Geometry check sheet. Reference: the model listing, model coordinates, mm. Face numbers are marked on the shaded views. A direction names the side the tool comes from. Give positions to 0.01 mm unless a question says otherwise; leave off trailing zeros. Loops run counter-clockwise (first coordinate to the right, second up) from the corner with the lowest first, then second, coordinate; pieces in that order, holes last. Notation, with made-up numbers: (76.25, 24.25) - (129.25, 24.25) arc R8 cw to (129.25, 30.25) - close; hole circle Ø8 at (36.25, -15). An arc over 180 degrees is marked (long way). Use a Markdown table: item, result. Add a question column.
1. Cross-section at A-A on z = 47. Enter the section's corners in (x, y), and give its area (3 significant figures).
2. Set-up check for the marked faces 1, 2, 3, 4 and 5: record each of +Z, -Z, +X, -X, +Y, -Y from which the full face is reachable in a straight line by a thin tool's end or side.
3. Depth check by flat-ended pin: P1, Ø3, axis at x = -51, y = 108.21, coming from the -Z side (3 decimals); P2, Ø4, axis at x = 31.5, z = 30, coming from the +Y side; P3, Ø10, axis at x = -39, z = 47, coming from the +Y side. Enter the tip coordinate at first touch or a pass-through.
4. Cross-section at B-B on x = 0. Enter the section's corners in (y, z), and give its area (3 significant figures).
5. Cross-section at C-C on z = 35.5. Enter the section's corners in (x, y).
6. Draft check along Y on the marked faces 6, 7 and 8. Enter one of: pulls with the +Y half, pulls with the -Y half, needs draft (parallel to the pull), parting line crosses it, or undercut.
7. Material ranges on L1, parallel to Y at x = 0, z = 2; L2, parallel to Y at x = 51, z = 4; L3, parallel to Z at x = 54.5, y = 77, recorded low to high.
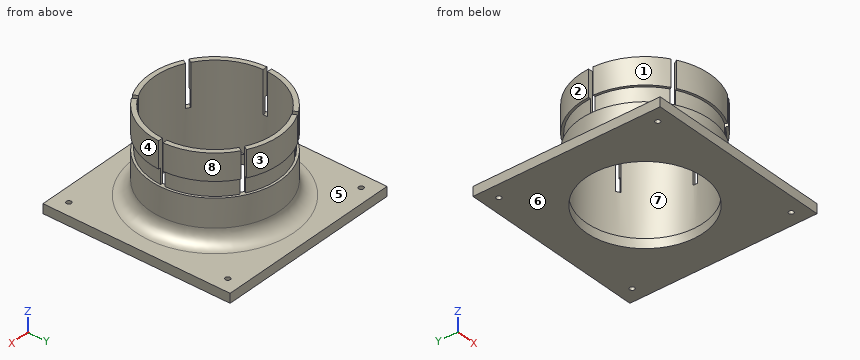
Autodesk Inventor part; units mm, degrees
ref_plane "Work Plane1" through (0, 57.2078, 33) normal (0, 0, 1) x (1, 0, 0)
ref_plane "YZ Plane" through (0, 0, 0) normal (1, 0, 0) x (0, 1, 0)
ref_plane "XZ Plane" through (0, 0, 0) normal (0, 1, 0) x (-1, 0, 0)
sketch "Sketch1" plane through (0, 0, 0) normal (0, 0, 1) x (1, 0, 0)
  circle A0 centre (-51, -113.7922) radius 1.55
  circle A1 centre (51, -113.7922) radius 1.55
  circle A2 centre (-51, 108.2078) radius 1.55
  circle A3 centre (51, 6.2078) radius 1.55
  circle A4 centre (51, 108.2078) radius 1.55
  circle A5 centre (-51, 6.2078) radius 1.55
  circle A6 centre (51, -11.7922) radius 1.55
  circle A7 centre (-51, -11.7922) radius 1.55
  circle A8 centre (0, -62.7922) radius 54
  circle A9 centre (0, 57.2078) radius 54
  line L0 (-60, 117.2078) -> (-60, -112.7922)
  arc A10 (-60, -112.7922) -> (-50, -122.7922) centre (-50, -112.7922) ccw
  line L1 (-50, -122.7922) -> (50, -122.7922)
  arc A11 (50, -122.7922) -> (60, -112.7922) centre (50, -112.7922) ccw
  line L2 (60, -112.7922) -> (60, 117.2078)
  line L3 (60, 117.2078) -> (-60, 117.2078)
  line L4 (-60, -2.7922) -> (60, -2.7922)
  line L5 (60, -2.7922) -> (60, 117.2078)
  line L6 (60, 117.2078) -> (-60, 117.2078)
  line L7 (-60, 117.2078) -> (-60, -2.7922)
  line L8 (-60, -2.7922) -> (60, 117.2078) construction
  line L9 (60, -2.7922) -> (-60, 117.2078) construction
  circle A12 centre (0, 57.2078) radius 37.5
  point P0 (0, 0)
  dimension "d3" = 75
extrude "Extrusion1" add sketch "Sketch1" along normal blind 6 contours A9 | L3 L2 L4 L0
sketch "Sketch3" plane through (0, 0, 6) normal (0, 0, 1) x (1, 0, 0)
  circle A0 centre (0, 57.2078) radius 37.5 construction
  circle A1 centre (0, 57.2078) radius 38.5
  circle A2 centre (0, 57.2078) radius 41.5
  point P0 (0, 0)
  dimension "d4" = 77
  dimension "d5" = 3
extrude "Extrusion2" add sketch "Sketch3" along normal blind 54
ref_plane "Work Plane1" through (0, 57.2078, 33) normal (0, 0, 1) x (1, 0, 0)
sketch "Sketch4" plane through (0, 57.2078, 33) normal (0, 0, 1) x (1, 0, 0)
  circle A0 centre (0, 0) radius 38.5 construction
  circle A1 centre (0, 0) radius 41.5
  circle A2 centre (0, 0) radius 40
  point P0 (0, -57.2078)
  dimension "d9" = 1.5
extrude "Extrusion3" cut sketch "Sketch4" along normal blind 10
sketch "Sketch5" plane through (0, 57.2078, 60) normal (0, 0, 1) x (1, 0, 0)
  circle A0 centre (0, 0) radius 38.5
  circle A1 centre (0, 0) radius 41.5
  line L0 (0, 0) -> (-53, 0) construction
  line L1 (0, 0) -> (-41.4747, -1.4483)
  circle A2 centre (0, 0) radius 41.5
  line L2 (0, 0) -> (-41.4747, 1.4483)
  point P0 (0, -57.2078)
  dimension "d12" = 4
extrude "Extrusion4" cut sketch "Sketch5" against normal up to surface (27 mm away) contours L2 L1 A0 | A0 L1 A1 L2 picked at (-25.658, -0.5972) picked at (-40.4973, 0.1493)
pattern_circular "Circular Pattern1" count 6 over 360 about axis through (0, 57.2078, 6) along (0, 0, 1) of "Extrusion4"
fillet "Fillet1" radius 9 1 edges at (-41.5, 57.2078, 6)
equation "\"d0\" = 2 * thickness"
equation "\"d5\" = thickness"
equation "\"d6\" = fixture_height"
equation "\"d9\" = 0.5 * thickness"
equation "\"d18\" = 3 * thickness"
equation "\"thickness\" = 3"
equation "\"fixture_height\" = 18 * thickness"
equation "\"d8\" = -0.5 * fixture_height"
properties part number "Cup_Dispenser_Fixture"
Values found:
| question | item | result |
|---|---|---|
| 1 | outline | (-41.47, 55.76) arc R41.5 ccw to (-21.99, 22.01) - (-20.4, 24.56) arc R38.5 cw to (-38.48, 55.86) - close; (-41.47, 58.66) - (-38.48, 58.55) arc R38.5 cw to (-20.4, 89.86) - (-21.99, 92.4) arc R41.5 ccw to start; (-19.48, 20.57) arc R41.5 ccw to (19.48, 20.57) - (18.07, 23.21) arc R38.5 cw to (-18.07, 23.21) - close; (-19.48, 93.85) - (-18.07, 91.2) arc R38.5 cw to (18.07, 91.2) - (19.48, 93.85) arc R41.5 ccw to start; (20.4, 24.56) - (21.99, 22.01) arc R41.5 ccw to (41.47, 55.76) - (38.48, 55.86) arc R38.5 cw to start; (20.4, 89.86) arc R38.5 cw to (38.48, 58.55) - (41.47, 58.66) arc R41.5 ccw to (21.99, 92.4) - close |
| 1 | area | 704 mm2 |
| 2 | face 1 | +Z, -X, -Y |
| 2 | face 2 | +Z, -X, +Y |
| 2 | face 3 | +Z, +Y |
| 2 | face 4 | +Z, +X, -Y |
| 2 | face 5 | +Z |
| 3 | P1 | passes through |
| 3 | P2 | stops at y = 86.4 |
| 3 | P3 | stops at y = 81 |
| 4 | outline | (-2.79, 0) - (19.71, 0) - (19.71, 6) - (18.71, 6) - (18.71, 60) - (15.71, 60) - (15.71, 43) - (17.21, 43) - (17.21, 33) - (15.71, 33) - (15.71, 15) arc R9 cw to (6.71, 6) - (-2.79, 6) - close; (94.71, 0) - (117.21, 0) - (117.21, 6) - (107.71, 6) arc R9 cw to (98.71, 15) - (98.71, 33) - (97.21, 33) - (97.21, 43) - (98.71, 43) - (98.71, 60) - (95.71, 60) - (95.71, 6) - (94.71, 6) - close |
| 4 | area | 599 mm2 |
| 5 | outline | (-39.98, 55.81) arc R40 ccw to (-21.2, 23.29) - (-20.4, 24.56) arc R38.5 cw to (-38.48, 55.86) - close; (-39.98, 58.6) - (-38.48, 58.55) arc R38.5 cw to (-20.4, 89.86) - (-21.2, 91.13) arc R40 ccw to start; (-18.78, 21.89) arc R40 ccw to (18.78, 21.89) - (18.07, 23.21) arc R38.5 cw to (-18.07, 23.21) - close; (-18.78, 92.53) - (-18.07, 91.2) arc R38.5 cw to (18.07, 91.2) - (18.78, 92.53) arc R40 ccw to start; (20.4, 24.56) - (21.2, 23.29) arc R40 ccw to (39.98, 55.81) - (38.48, 55.86) arc R38.5 cw to start; (20.4, 89.86) arc R38.5 cw to (38.48, 58.55) - (39.98, 58.6) arc R40 ccw to (21.2, 91.13) - close |
| 6 | face 6 | needs draft |
| 6 | face 7 | undercut |
| 6 | face 8 | pulls with the +Y half |
| 7 | L1 | y = -2.79 to 19.71, 94.71 to 117.21 |
| 7 | L2 | y = -2.79 to 4.66, 7.76 to 106.66, 109.76 to 117.21 |
| 7 | L3 | z = 0 to 6 |
